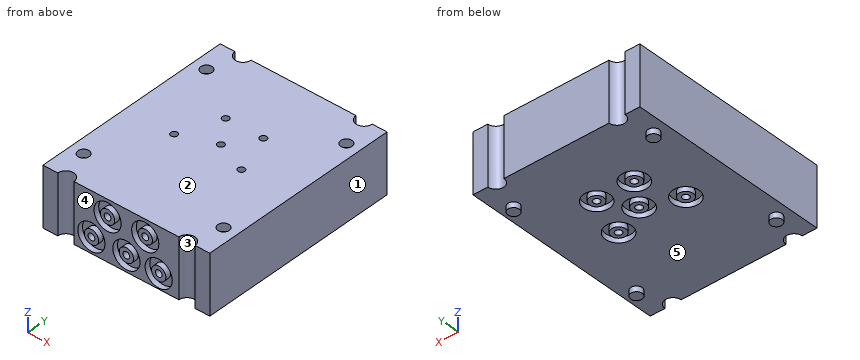
```python
from build123d import *

# Parameters (mm, degrees)
F0_W      = 62
F0_H      = 75
F1_DEPTH  = 14
F2_W      = 62
F2_H      = 75
F3_DEPTH  = 8
F4_R      = 1.25
F5_DEPTH  = 38
F6_R      = 4.85
F6_R_2    = 2.65
F7_DEPTH  = 2
F9_R      = 1.25
F10_DEPTH = 50
F11_R     = 5.05
F11_R_2   = 2.65
F12_DEPTH = 2
F13_DEPTH = 40
F14_DEPTH = 34.6
F16_DEPTH = 22
F8_R      = 2.1
F17_DEPTH = 3
F18_R     = 2.1
F19_DEPTH = 2


with BuildPart() as f1:
    # F0 (on Top) → F1 (new body)
    with BuildSketch(Plane.XY):
        Rectangle(F0_W, F0_H)
    extrude(amount=F1_DEPTH)

    # F2 (on face) → F3 (join)
    with BuildSketch(Plane(origin=(0, 0, 0), x_dir=(1, 0, 0), z_dir=(0, 0, -1))):
        Rectangle(F2_W, F2_H)
    extrude(amount=F3_DEPTH)

    # F4 (on face) → F5 (cut)
    with BuildSketch(Plane(origin=(0, 0, -8), x_dir=(1, 0, 0), z_dir=(0, 0, -1))):
        with Locations((-13, 2.5)):
            Circle(F4_R)
        with Locations((-7, -12.5)):
            Circle(F4_R)
        with Locations((0, -2.5)):
            Circle(F4_R)
        with Locations((7, -12.5)):
            Circle(F4_R)
        with Locations((12, 2.5)):
            Circle(F4_R)
    extrude(amount=-F5_DEPTH, mode=Mode.SUBTRACT)

    # F6 (on face) → F7 (cut)
    with BuildSketch(Plane(origin=(0, 0, -8), x_dir=(1, 0, 0), z_dir=(0, 0, -1))):
        with Locations((-7, -12.5)):
            Circle(F6_R)
        with Locations((-7, -12.5)):
            Circle(F6_R_2, mode=Mode.SUBTRACT)
        with Locations((-13, 2.5)):
            Circle(F6_R)
        with Locations((-13, 2.5)):
            Circle(F6_R_2, mode=Mode.SUBTRACT)
        with Locations((0, -2.5)):
            Circle(F6_R)
        with Locations((0, -2.5)):
            Circle(F6_R_2, mode=Mode.SUBTRACT)
        with Locations((12, 2.5)):
            Circle(F6_R)
        with Locations((12, 2.5)):
            Circle(F6_R_2, mode=Mode.SUBTRACT)
        with Locations((7, -12.5)):
            Circle(F6_R)
        with Locations((7, -12.5)):
            Circle(F6_R_2, mode=Mode.SUBTRACT)
    extrude(amount=-F7_DEPTH, mode=Mode.SUBTRACT)

    # F9 (on face) → F10 (cut)
    with BuildSketch(Plane.XZ.offset(37.5)):
        with Locations((-7, 7.8316577617)):
            Circle(F9_R)
        with Locations((7, 7.8316577617)):
            Circle(F9_R)
    extrude(amount=-F10_DEPTH, mode=Mode.SUBTRACT)

    # F11 (on face) → F12 (cut)
    with BuildSketch(Plane.XZ.offset(37.5)):
        with Locations((-7, 7.8316577617)):
            Circle(F11_R)
        with Locations((-7, 7.8316577617)):
            Circle(F11_R_2, mode=Mode.SUBTRACT)
        with Locations((-13, -2.1683422383)):
            Circle(F11_R)
        with Locations((-13, -2.1683422383)):
            Circle(F11_R_2, mode=Mode.SUBTRACT)
        with Locations((0, -2.0990659878)):
            Circle(F11_R)
        with Locations((0, -2.0990659878)):
            Circle(F11_R_2, mode=Mode.SUBTRACT)
        with Locations((12, -2.5362078735)):
            Circle(F11_R)
        with Locations((12, -2.5362078735)):
            Circle(F11_R_2, mode=Mode.SUBTRACT)
        with Locations((7, 7.8316577617)):
            Circle(F11_R)
        with Locations((7, 7.8316577617)):
            Circle(F11_R_2, mode=Mode.SUBTRACT)
    extrude(amount=-F12_DEPTH, mode=Mode.SUBTRACT)

    # F9 (on face) → F13 (cut)
    with BuildSketch(Plane.XZ.offset(37.5)):
        with Locations((0, -2.0990659878)):
            Circle(F9_R)
    extrude(amount=-F13_DEPTH, mode=Mode.SUBTRACT)

    # F9 (on face) → F14 (cut)
    with BuildSketch(Plane.XZ.offset(37.5)):
        with Locations((12, -2.5362078735)):
            Circle(F9_R)
        with Locations((-13, -2.1683422383)):
            Circle(F9_R)
    extrude(amount=-F14_DEPTH, mode=Mode.SUBTRACT)

    # F15 (on face) → F16 (cut)
    with BuildSketch(Plane(origin=(0, 0, -8), x_dir=(1, 0, 0), z_dir=(0, 0, -1))):
        with BuildLine():
            ThreePointArc((-25.5, 37.5), (-22.5, 34.5), (-19.5, 37.5))
            Line((-19.5, 37.5), (-25.5, 37.5))
        make_face()
        with BuildLine():
            Line((25.5, 37.5), (19.5, 37.5))
            ThreePointArc((19.5, 37.5), (22.5, 34.5), (25.5, 37.5))
        make_face()
        with BuildLine():
            ThreePointArc((-19.5, -37.5), (-22.5, -34.5), (-25.5, -37.5))
            Line((-25.5, -37.5), (-19.5, -37.5))
        make_face()
        with BuildLine():
            Line((19.5, -37.5), (25.5, -37.5))
            ThreePointArc((25.5, -37.5), (22.5, -34.5), (19.5, -37.5))
        make_face()
    extrude(amount=-F16_DEPTH, mode=Mode.SUBTRACT)

    # F8 (on face) → F17 (cut)
    with BuildSketch(Plane.XY.offset(14)):
        with Locations((-26, 26)):
            Circle(F8_R)
        with Locations((-26, -26)):
            Circle(F8_R)
        with Locations((26, -26)):
            Circle(F8_R)
        with Locations((26, 26)):
            Circle(F8_R)
    extrude(amount=-F17_DEPTH, mode=Mode.SUBTRACT)

    # F18 (on face) → F19 (join)
    with BuildSketch(Plane(origin=(0, 0, -8), x_dir=(1, 0, 0), z_dir=(0, 0, -1))):
        with Locations((-26, 26)):
            Circle(F18_R)
        with Locations((26, 26)):
            Circle(F18_R)
        with Locations((26, -26)):
            Circle(F18_R)
        with Locations((-26, -26)):
            Circle(F18_R)
    extrude(amount=F19_DEPTH)


solid = f1.part
```
The listing builds one solid part. Answer for the finished solid, in the listing's coordinates (mm). Face numbers are marked on the shaded views. A direction names the side the tool comes from. Round coordinates to 2 decimals unless told otherwise and drop trailing zeros. Loops run counter-clockwise (first coordinate to the right, second up) from the corner with the lowest first, then second, coordinate; pieces in that order, holes last.
Q1. Section C-C, the plane y = -13 is taken. Determine the outline of the cut face in (x, z).
Q2. Find the intervals of material crossed by line 1 (Y direction, x = -26, z = 11.7); line 2 (Y direction, x = -13, z = -6.6); line 3 (Y direction, x = -13, z = 4), in increasing order.
Q3. Which of the six approach directions +Z, -Z, +X, -X, +Y, -Y give full straight-line access (tool end or side, diameter ignored) to the marked faces 4 and 5?
Q4. Section B-B, the plane y = 26 is taken. Determine the outline of the cut face in (x, z).
Q5. For a pull along X with two mould halves and no side action, classify the marked faces 1, 2 and 3 as released by +X, released by -X, zero draft, split by the parting line, or undercut.
Q6. Given pin 1 Ø3 at (x, y) = (14.5, -0.5) entering from -Z; pin 2 Ø3 at (x, z) = (12, -2.54) entering from -Y; pin 3 Ø1.3 at (x, y) = (25.5, -25) entering from +Z; pin 4 Ø1 at (x, z) = (20.5, 3.5) entering from -Y, each flat-ended and moving along its own axis, determine where each tip first touches the part or whether it passes through.
Q7. Section D-D, the plane x = 0 is taken. Determine the outline of the cut face in (y, z).
Q8. Section A-A, the plane x = -13 is taken. Determine the outline of the cut face in (y, z), then the cut area to 3 significant figures.
Completed:
1. outline: (-31, -8) - (31, -8) - (31, 14) - (-31, 14) - close; hole circle Ø2.5 at (-13, -2.17); hole circle Ø2.5 at (-7, 7.83); hole circle Ø2.5 at (0, -2.1); hole circle Ø2.5 at (7, 7.83); hole circle Ø2.5 at (12, -2.54)
2. line 1: y = -37.5 to -28.1, -23.9 to 23.9, 28.1 to 37.5
2. line 2: y = -35.5 to -7.35, -5.15 to -3.75, -1.25 to 0.15, 2.35 to 37.5
2. line 3: y = -37.5 to -3.75, -1.25 to 37.5
3. face 4: +Z, -Z, +X, -X, -Y
3. face 5: -Z
4. outline: (-31, -8) - (-28.1, -8) - (-28.1, -10) - (-23.9, -10) - (-23.9, -8) - (23.9, -8) - (23.9, -10) - (28.1, -10) - (28.1, -8) - (31, -8) - (31, 14) - (28.1, 14) - (28.1, 11) - (23.9, 11) - (23.9, 14) - (-23.9, 14) - (-23.9, 11) - (-28.1, 11) - (-28.1, 14) - (-31, 14) - close
5. face 1: released by +X
5. face 2: zero draft
5. face 3: undercut
6. pin 1: stops at z = -8
6. pin 2: stops at y = -37.5
6. pin 3: stops at z = 11
6. pin 4: stops at y = -35.84
7. outline: (-37.5, -8) - (-2.35, -8) - (-2.35, -6) - (-0.15, -6) - (-0.15, -8) - (1.25, -8) - (1.25, -3.35) - (-37.5, -3.35) - (-37.5, -4.75) - (-35.5, -4.75) - (-35.5, -7.15) - (-37.5, -7.15) - close; (-37.5, -0.85) - (1.25, -0.85) - (1.25, 14) - (-37.5, 14) - (-37.5, 2.95) - (-35.5, 2.95) - (-35.5, 0.55) - (-37.5, 0.55) - close; (3.75, -8) - (5.15, -8) - (5.15, -6) - (7.35, -6) - (7.35, -8) - (37.5, -8) - (37.5, 14) - (3.75, 14) - close
8. outline: (-37.5, -8) - (-7.35, -8) - (-7.35, -6) - (-5.15, -6) - (-5.15, -8) - (-3.75, -8) - (-3.75, -3.42) - (-37.5, -3.42) - (-37.5, -4.82) - (-35.5, -4.82) - (-35.5, -7.22) - (-37.5, -7.22) - close; (-37.5, -0.92) - (-3.75, -0.92) - (-3.75, 14) - (-37.5, 14) - (-37.5, 2.88) - (-35.5, 2.88) - (-35.5, 0.48) - (-37.5, 0.48) - close; (-1.25, -8) - (0.15, -8) - (0.15, -6) - (2.35, -6) - (2.35, -8) - (37.5, -8) - (37.5, 14) - (-1.25, 14) - close
8. area: 1,490 mm2
